Build history of the part. All positions in model axes, mm. A direction names the side the tool comes from. Round coordinates to 2 decimals unless told otherwise and drop trailing zeros. Order: outer loops, then holes, each group sorted by start corner. A loop starts at its lowest first (then second) coordinate and runs counter-clockwise, first axis right, second up. Notation, with made-up numbers: M 5.25,88 L 44.25,88 A14 ccw 44.25,106 Z; hole C 50,72.5 d4. An arc over 180 degrees is marked long. Use CSV: the item, a comma, the result in double quotes.
from build123d import *

# Parameters (mm, degrees)
PAD_DEPTH       = 41
SKETCH001_W     = 106.614
SKETCH001_H     = 35
POCKET_DEPTH    = 27.7
SKETCH002_R     = 10
SKETCH002_R_2   = 1.75
POCKET001_DEPTH = 41.001
SKETCH003_R     = 14
POCKET002_DEPTH = 31.701
SKETCH004_R     = 6
POCKET003_DEPTH = 114.865


with BuildPart() as part:
    # Sketch → Pad (new body)
    with BuildSketch(Plane.XY):
        with BuildLine():
            Line((-60.41588, 16.2), (52.19812, 16.2))
            Line((52.19812, 16.2), (52.19812, -13.517735))
            ThreePointArc((45.538339, -15.5), (50.967872, -21.563001), (52.19812, -13.517735))
            Line((-53.5, -15.5), (45.538339, -15.5))
            ThreePointArc((-60.41588, -13.211126), (-59.408323, -21.759447), (-53.5, -15.5))
            Line((-60.41588, -13.211126), (-60.41588, 16.2))
        make_face()
    extrude(amount=PAD_DEPTH)

    # Sketch001 → Pocket (cut)
    with BuildSketch(Plane(origin=(0, 16.2, 0), x_dir=(-1, 0, 0), z_dir=(0, 1, 0))):
        with Locations((4.10888, 20.5)):
            Rectangle(SKETCH001_W, SKETCH001_H)
    extrude(amount=-POCKET_DEPTH, mode=Mode.SUBTRACT)

    # Sketch002 → Pocket001 (cut, through all)
    with BuildSketch(Plane.XY.offset(41)):
        with Locations((-31.91588, 0)):
            Circle(SKETCH002_R)
        Circle(SKETCH002_R)
        with Locations((30, 0)):
            Circle(SKETCH002_R)
        with Locations((49.938726, -17.458258)):
            Circle(SKETCH002_R_2)
        with Locations((-57.661274, -17.584375)):
            Circle(SKETCH002_R_2)
        with BuildLine():
            ThreePointArc((-57.41588, -7.499976), (-52.415893, -12.499999), (-47.41588, -7.5))
            Line((-47.41588, -7.5), (-47.41588, 8.2))
            ThreePointArc((-47.41588, 8.2), (-52.41587, 13.2), (-57.41588, 8.200022))
            Line((-57.41588, -7.499976), (-57.41588, 8.200022))
        make_face()
    extrude(amount=-POCKET001_DEPTH, mode=Mode.SUBTRACT)

    # Sketch003 → Pocket002 (cut, through all)
    with BuildSketch(Plane.XZ.offset(15.5)):
        with Locations((-28.5, 20)):
            Circle(SKETCH003_R)
        with Locations((20.538339, 20)):
            Circle(SKETCH003_R)
    extrude(amount=-POCKET002_DEPTH, mode=Mode.SUBTRACT)

    # Sketch004 → Pocket003 (cut, through all)
    with BuildSketch(Plane.YZ.offset(52.19812)):
        with Locations((0, 30.5)):
            Circle(SKETCH004_R)
        with Locations((0, 10.5)):
            Circle(SKETCH004_R)
    extrude(amount=-POCKET003_DEPTH, mode=Mode.SUBTRACT)


solid = part.part
(1) Wall check: line 1 (Z direction, x = 50.75, y = 0); line 2 (Z direction, x = -46, y = 0.5); line 3 (X direction, y = -7, z = 9.5). Give the ranges that are in metal, low to high. Write a range as from..to.
Answer block:
line 1,"z = 0..4.5, 16.5..24.5, 36.5..41"
line 2,"z = 0..3, 38..41"
line 3,"x = -60.42..-57.42, 49.2..52.2"
(2) Tool access for faces 4 (the face through (50.719, -1.301, 24.643)), 5 (the face through (-56, -11.5, 21)), 6 (the face through (-47.416, 0, 40)): list every direction of +Z, -Z, +X, -X, +Y, -Y with a clear straight run to the whole face (end or side of a thin tool).
Answer block:
face 4,"+X, -X"
face 5,"+Y"
face 6,"+Z, -Z"
(3) Two-plate mould, pull along X, no slides. Class faces 1 (the face through (-3, -11, 41)), 2 (the face through (-41.906, 0.44, 1.521)), 3 (the face through (-60.416, 1, 20)): released by +X, released by -X, zero draft, split by the parting line, or undercut.
Answer block:
face 1,"zero draft"
face 2,"undercut"
face 3,"released by -X"
(4) Cut at D-D, the plane x = -28.5. Give the cut face in (y, z), and give its area (3 significant figures).
Answer block:
outline,"M -15.5,0 L -9.4,0 L -9.4,3 L -11.5,3 L -11.5,6 L -15.5,6 Z; M -15.5,34 L -11.5,34 L -11.5,38 L -9.4,38 L -9.4,41 L -15.5,41 Z; M 9.4,0 L 16.2,0 L 16.2,3 L 9.4,3 Z; M 9.4,38 L 16.2,38 L 16.2,41 L 9.4,41 Z"
area,"105 mm²"
(5) Cut at C-C, the plane z = 20. Give the cut face in (x, y), and give its area (3 significant figures).
Answer block:
outline,"M -60.42,-13.21 A4.75 ccw long -53.5,-15.5 L -42.5,-15.5 L -42.5,-11.5 L -49.42,-11.5 A5 cw -55.42,-11.5 L -57.42,-11.5 L -57.42,16.2 L -60.42,16.2 Z; M -14.5,-15.5 L 6.54,-15.5 L 6.54,-11.5 L -14.5,-11.5 Z; M 34.54,-15.5 L 45.54,-15.5 A4.5 ccw long 52.2,-13.52 L 52.2,16.2 L 49.2,16.2 L 49.2,-11.5 L 34.54,-11.5 Z; hole C -57.66,-17.58 d3.5; hole C 49.94,-17.46 d3.5"
area,"473 mm²"
(6) Cut at B-B, the plane z = 13.5. Count the separate pieces of the cut face and the enclosed holes in it, and give its area (3 significant figures).
Answer block:
separate pieces,"5"
enclosed holes,"2"
area,"436 mm²"
(7) Cut at A-A, the plane x = 36. Give the cut face in (y, z).
Answer block:
outline,"M -15.5,0 L -8,0 L -8,3 L -11.5,3 L -11.5,38 L -8,38 L -8,41 L -15.5,41 Z; M 8,0 L 16.2,0 L 16.2,3 L 8,3 Z; M 8,38 L 16.2,38 L 16.2,41 L 8,41 Z"
(8) Drop flat-ended pins along their axis: pin 1 (1.6 mm diameter, centred on x = -57, y = -9, fed in from +Z); pin 2 (22 mm diameter, centred on y = -0.5, z = 25, fed in from +X); pin 3 (10 mm diameter, centred on y = -9, z = 15.5, fed in from -X); pin 4 (2.5 mm diameter, centred on y = -1.5, z = 39, fed in from -X). Give the stop position or say it passes through.
Answer block:
pin 1,"stops at z = 41"
pin 2,"stops at x = 52.2"
pin 3,"stops at x = -61.38"
pin 4,"stops at x = -60.42"
